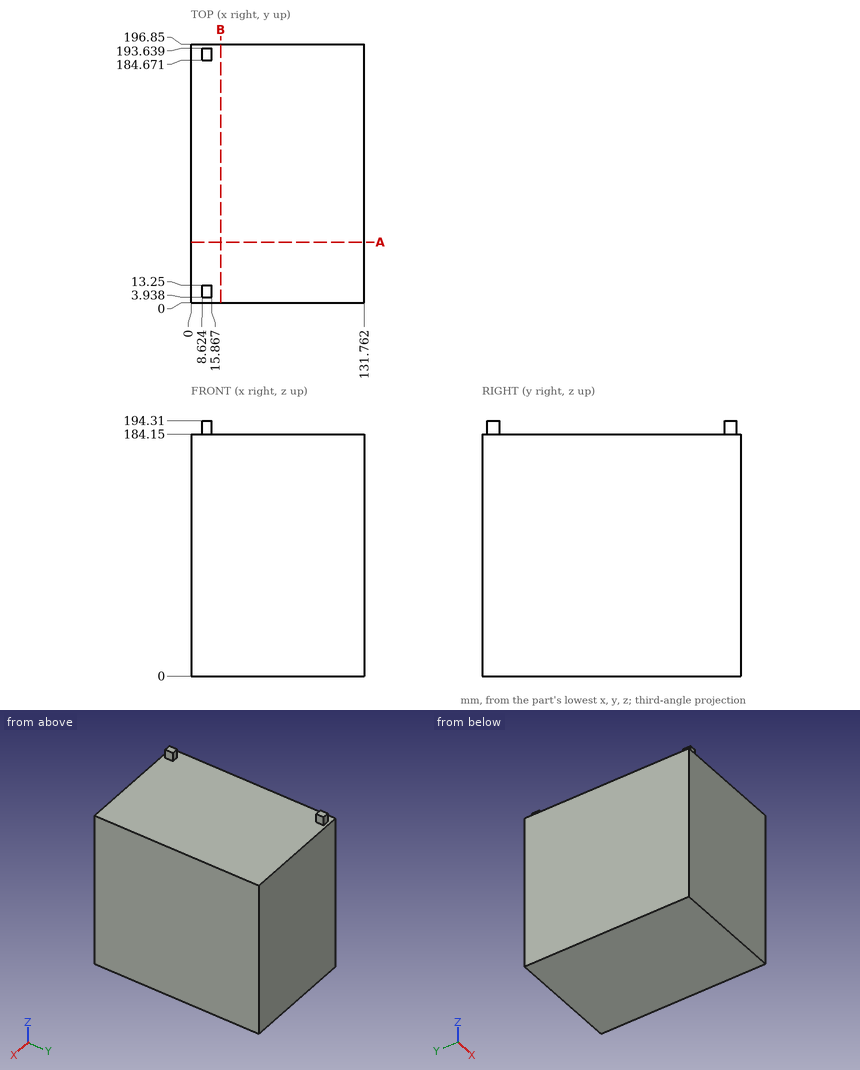
Source: three-view drawing plus pictorial views. Frame: mm from the lowest corner of the part. Round coordinates to 2 decimals unless told otherwise and drop trailing zeros. Loops run counter-clockwise (first coordinate to the right, second up) from the corner with the lowest first, then second, coordinate; pieces in that order, holes last.
Q1. Material intervals for L1, parallel to Z at x = 24, y = 70, sorted ascending.
Q2. Section B-B on x = 22.5. Return loops of the section in (y, z).
Q3. Section A-A on y = 46. Return loops of the section in (x, z).
Q4. Pin query (flat end, axial travel): P1, Ø7, axis at y = 189.5, z = 190.5, coming from the -X side; P2, Ø6, axis at x = 14, z = 189, coming from the +Y side; P3, Ø4.5, axis at y = 190.5, z = 191, coming from the +X side; P4, Ø3, axis at y = 35, z = 61.5, coming from the -X side. Return the tip coordinate at first contact, or that it passes through.
Evaluation:
1. L1: z = 0 to 184.15
2. outline: (0, 0) - (196.85, 0) - (196.85, 184.15) - (0, 184.15) - close
3. outline: (0, 0) - (131.76, 0) - (131.76, 184.15) - (0, 184.15) - close
4. P1: stops at x = 8.62
4. P2: stops at y = 193.64
4. P3: stops at x = 15.87
4. P4: stops at x = 0
